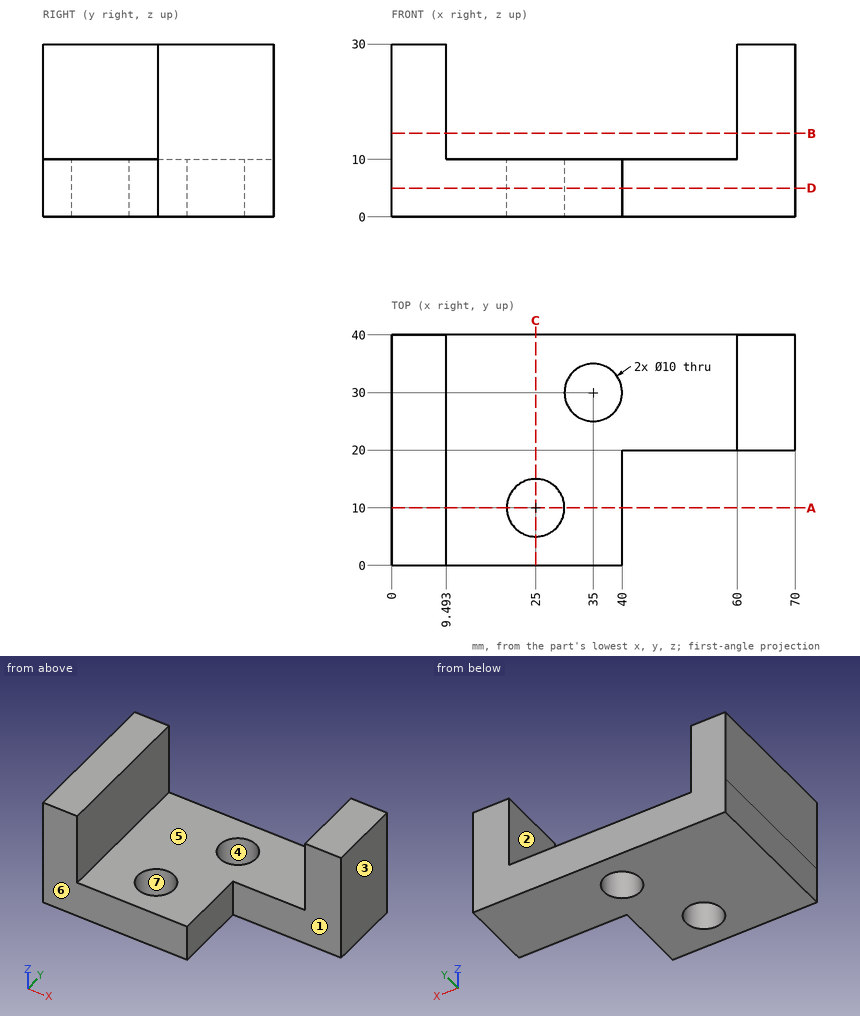
Study the drawing (mm; zero at the part's minimum x, y, z) and answer. A direction names the side the tool comes from. Give positions to 0.01 mm unless a question says otherwise; leave off trailing zeros. Order: outer loops, then holes, each group sorted by start corner. A loop starts at its lowest first (then second) coordinate and runs counter-clockwise, first axis right, second up. Notation, with made-up numbers: (1, 0) - (47, 0) arc R16 ccw to (47, 11) - close; hole circle Ø1 at (77, 20.25). An arc over 180 degrees is marked (long way). Use one line per item in the form item = value. Start each with the question number.
(1) Flat-ended cylindrical pins translate along their axes: pin 1 Ø8 at (x, z) = (27, 16) entering from -Y; pin 2 Ø4 at (x, y) = (15.5, 29) entering from +Z; pin 3 Ø5 at (y, z) = (7, 5) entering from +X; pin 4 Ø2 at (y, z) = (6.5, 23) entering from +X. Find the tip coordinate at first contact, or state that the pin passes through.
(2) A cutting plane is placed at B-B, the plane z = 14.5. Write down the section's boundary in (x, y).
(3) A cutting plane is placed at A-A, the plane y = 10. Write down the section's boundary in (x, z).
(4) Consider line 1 (X direction, y = 33.5, z = 17.5); line 2 (Y direction, x = 35, z = 7.75); line 3 (Z direction, x = 45, y = 27). Determine where each line is inside the solid, lowest interval first. Write a range as from..to.
(5) The mould has two halves that part along Y. Classify the marked faces 4, 5, 6 and 7: released by +Y, released by -Y, zero draft, split by the parting line, or undercut.
(6) For the marked faces 1, 2 and 3, determine the directions among +Z, -Z, +X, -X, +Y, -Y from which every point of the face is accessible in a straight line to the end or side of a thin tool.
(7) A cutting plane is placed at D-D, the plane z = 5. Write down the section's boundary in (x, y).
(8) A cutting plane is placed at C-C, the plane x = 25. Write down the section's boundary in (y, z), then the cut area to 3 significant figures.
Ans:
q1.pin_1 = through
q1.pin_2 = 10
q1.pin_3 = 40
q1.pin_4 = 9.49
q2.outline = (0, 0) - (9.49, 0) - (9.49, 40) - (0, 40) - close; (60, 20) - (70, 20) - (70, 40) - (60, 40) - close
q3.outline = (0, 0) - (20, 0) - (20, 10) - (9.49, 10) - (9.49, 30) - (0, 30) - close; (30, 0) - (40, 0) - (40, 10) - (30, 10) - close
q4.line_1 = 0..9.49, 60..70
q4.line_2 = 0..25, 35..40
q4.line_3 = 0..10
q5.face_4 = undercut
q5.face_5 = zero draft
q5.face_6 = released by -Y
q5.face_7 = undercut
q6.face_1 = +Z, -Z, +X, -Y
q6.face_2 = +Z, +Y, -Y
q6.face_3 = +Z, -Z, +X, +Y, -Y
q7.outline = (0, 0) - (40, 0) - (40, 20) - (70, 20) - (70, 40) - (0, 40) - close; hole circle Ø10 at (25, 10); hole circle Ø10 at (35, 30)
q8.outline = (0, 0) - (5, 0) - (5, 10) - (0, 10) - close; (15, 0) - (40, 0) - (40, 10) - (15, 10) - close
q8.area = 300 mm^2
